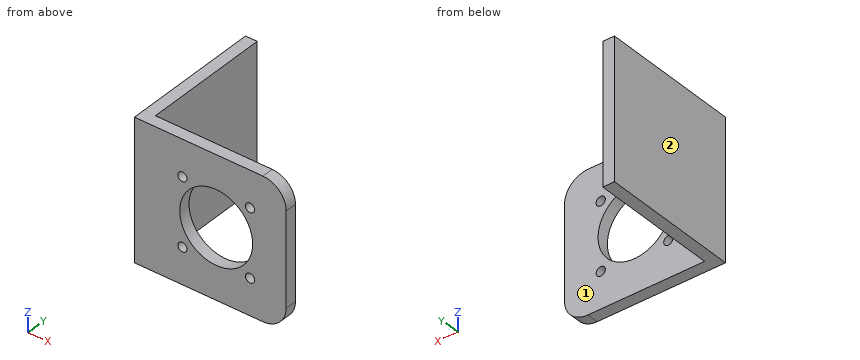
from build123d import *

# Parameters (mm, degrees)
F1_DEPTH = 38.1
F2_R     = 9.921835
F2_R_2   = 1.25
F3_DEPTH = 3.175
F4_R     = 6.35


with BuildPart() as f1:
    # F0 (on Top) → F1 (new body)
    with BuildSketch(Plane.XY):
        Polygon((0, 38.1), (0, 0), (41.275, 0), (41.275, 3.175), (3.175, 3.175), (3.175, 38.1), align=None)
    extrude(amount=F1_DEPTH)

    # F2 (on face) → F3 (cut, through all)
    with BuildSketch(Plane(origin=(0, 3.175, 0), x_dir=(-1, 0, 0), z_dir=(0, 1, 0))):
        with Locations((-22.225, 19.05)):
            Circle(F2_R)
        with Locations((-13.032612, 9.857612)):
            Circle(F2_R_2)
        with Locations((-31.417388, 28.242388)):
            Circle(F2_R_2)
        with Locations((-31.417388, 9.857612)):
            Circle(F2_R_2)
        with Locations((-13.032612, 28.242388)):
            Circle(F2_R_2)
    extrude(amount=-F3_DEPTH, mode=Mode.SUBTRACT)

    # F4
    f4_edges = [f1.edges().sort_by_distance(p)[0] for p in [
        (41.275, 1.5875, 38.1),
        (41.275, 1.5875, 0),
    ]]
    fillet(f4_edges, radius=F4_R)


solid = f1.part
Model file for the job. Use its own axes, mm. Face numbers are marked on the shaded views. A direction names the side the tool comes from. Round coordinates to 2 decimals unless told otherwise and drop trailing zeros. Order: outer loops, then holes, each group sorted by start corner. A loop starts at its lowest first (then second) coordinate and runs counter-clockwise, first axis right, second up.
(1) Band-saw the part on A-A (z = 19.05). List the corners of the cut face in (x, y) (3 decimals), then the cut area to 3 significant figures.
(2) Drill centre lines: line 1 (X direction, y = 1, z = 19) (3 decimals); line 2 (X direction, y = 11, z = 28.5) (3 decimals). Where is each one in solid material? Low to high.
(3) Band-saw the part on B-B (x = 27.5). List the corners of the cut face in (y, z) (3 decimals).
(4) Band-saw the part on C-C (z = 7). List the corners of the cut face in (x, y) (3 decimals).
(5) Band-saw the part on D-D (y = 29). List the corners of the cut face in (x, z) (3 decimals), then the cut area to 3 significant figures.
(6) Pin check, flat tips, straight feed: pin 1 (3 mm diameter, centred on x = 31.42, z = 9.86, fed in from +Y) (3 decimals); pin 2 (3 mm diameter, centred on y = 22, z = 10, fed in from +X) (3 decimals); pin 3 (12 mm diameter, centred on x = 22.225, z = 19.05, fed in from +Y). Stop position of each tip, or through.
(7) 3-axis set-ups, long thin cutter, end or side, ignore diameter. For the marked faces 1 and 2: which of +Z, -Z, +X, -X, +Y, -Y reach the whole face in a straight line?
Verdict:
1. outline: (0, 0) - (12.303, 0) - (12.303, 3.175) - (3.175, 3.175) - (3.175, 38.1) - (0, 38.1) - close; (32.147, 0) - (41.275, 0) - (41.275, 3.175) - (32.147, 3.175) - close
1. area: 179 mm2
2. line 1: x = 0 to 12.303, 32.147 to 41.275
2. line 2: x = 0 to 3.175
3. outline: (0, 0) - (3.175, 0) - (3.175, 10.647) - (0, 10.647) - close; (0, 27.453) - (3.175, 27.453) - (3.175, 38.1) - (0, 38.1) - close
4. outline: (0, 0) - (41.275, 0) - (41.275, 3.175) - (3.175, 3.175) - (3.175, 38.1) - (0, 38.1) - close
5. outline: (0, 0) - (3.175, 0) - (3.175, 38.1) - (0, 38.1) - close
5. area: 121 mm2
6. pin 1: stops at y = 3.175
6. pin 2: stops at x = 3.175
6. pin 3: passes through
7. face 1: +Z, -Z, +X, +Y
7. face 2: +Z, -Z, -X, +Y, -Y
